CAD build for the part. Positions are in the model's coordinates, mm. A direction names the side the tool comes from. Coordinates: 2 decimals unless noted, no trailing zeros. Loops run counter-clockwise (first coordinate to the right, second up) from the corner with the lowest first, then second, coordinate; pieces in that order, holes last. Notation, with made-up numbers: (82, -19) - (116, -19) arc R25 cw to (116, 4) - close; hole circle Ø11 at (2, 49). An arc over 180 degrees is marked (long way). Put each result on its own line as item: value.
Autodesk Inventor part; units mm, degrees
ref_plane "Work Plane1" through (0, 0, -15) normal (0, 0, 1) x (1, 0, 0)
ref_plane "YZ Plane" through (0, 0, 0) normal (1, 0, 0) x (0, 1, 0)
ref_plane "XZ Plane" through (0, 0, 0) normal (0, 1, 0) x (-1, 0, 0)
sketch "Sketch1" plane through (0, 0, 0) normal (0, 0, 1) x (1, 0, 0)
  line L0 (0, 0) -> (25, 0)
  line L1 (25, 0) -> (25, 40)
  line L2 (25, 40) -> (0, 40)
  line L3 (0, 40) -> (0, 0)
  dimension "d1" = 25
  dimension "d2" = 40
  dimension "d3" = 25
extrude "Extrusion1" add sketch "Sketch1" against normal blind 30
sketch "Sketch2" plane through (25, 0, 0) normal (1, 0, 0) x (0, 0, -1)
  line L0 (0, 0) -> (30, 0)
  circle A0 centre (15, 6.56) radius 2.46
extrude "Extrusion2" cut sketch "Sketch2" against normal blind 30
sketch "Sketch3" plane through (0, 0, 0) normal (-1, 0, 0) x (0, 0, 1)
  line L0 (0, 0) -> (-30, 0)
  line L1 (-25.05, 0) -> (-4.95, 0)
  line L2 (-4.95, 0) -> (-4.95, 33.12)
  line L3 (-4.95, 33.12) -> (-25.05, 33.12)
  line L4 (-25.05, 33.12) -> (-25.05, 0)
  dimension "d11" = 20.1
extrude "Extrusion3" cut sketch "Sketch3" against normal blind 20
sketch "Sketch4" plane through (0, 0, 0) normal (0, -1, 0) x (1, 0, 0)
  line L0 (20, -4.95) -> (20, -25.05)
  line L1 (20, -15) -> (25, -15)
  line L2 (25, 0) -> (25, -30)
  line L3 (20, -8.025) -> (25, -8.025)
  line L4 (25, -8.025) -> (25, -21.975)
  line L5 (25, -21.975) -> (20, -21.975)
  line L6 (20, -21.975) -> (20, -8.025)
  line L7 (20, -8.025) -> (25, -21.975) construction
  line L8 (25, -8.025) -> (20, -21.975) construction
  line L9 (25, -12.54) -> (25, -17.46)
  point P0 (0, 0)
  point P1 (22.5, -15)
  dimension "d14" = 13.95
extrude "Extrusion4" add sketch "Sketch4" along normal blind 15
sketch "Sketch5" plane through (20, 0, 0) normal (-1, 0, 0) x (0, 0, 1)
  circle A0 centre (-15, 6.56) radius 2.46
  circle A1 centre (-15, 6.56) radius 4.7025
  circle A2 centre (-15, 6.56) radius 2.46
  circle A3 centre (-15, 6.56) radius 2.46
  point P0 (0, 0)
  dimension "d17" = 9.405
extrude "Extrusion5" cut sketch "Sketch5" against normal blind 2.1
sketch "Sketch6" plane through (25, 0, 0) normal (1, 0, 0) x (0, 0, -1)
  circle A0 centre (15, 6.56) radius 4.7025
  line L0 (15, 6.56) -> (15, 23.56)
  circle A1 centre (15, 23.56) radius 2.46
  point P0 (0, 0)
  dimension "d20" = 17
  dimension "d21" = 4.92
extrude "Extrusion6" cut sketch "Sketch6" against normal blind 10 contours A1
sketch "Sketch7" plane through (20, 0, 0) normal (-1, 0, 0) x (0, 0, 1)
  circle A0 centre (-15, 23.56) radius 2.46
  circle A1 centre (-15, 23.56) radius 4.7025
  point P0 (0, 0)
  dimension "d24" = 9.405
extrude "Extrusion7" cut sketch "Sketch7" against normal blind 2.1
sketch "Sketch9" plane through (25, 0, 0) normal (1, 0, 0) x (0, 0, -1)
  circle A0 centre (15, 6.56) radius 2.46
  circle A1 centre (15, 6.56) radius 2.46
  circle A2 centre (15, 23.56) radius 2.46
  circle A3 centre (15, 23.56) radius 2.46
  line L0 (30, 40) -> (30, 0)
  line L1 (30, 0) -> (30, 40)
  line L2 (30, 40) -> (0, 40)
  line L3 (0, 40) -> (0, 0)
  line L4 (0, 0) -> (8.025, 0)
  line L5 (21.975, 0) -> (21.975, -15)
  line L6 (21.975, -15) -> (8.025, -15)
  line L7 (8.025, -15) -> (8.025, 0)
  line L8 (0, 0) -> (8.025, 0)
  line L9 (21.975, 0) -> (30, 0)
extrude "Extrusion8" add sketch "Sketch9" along normal blind 5
sketch "Sketch10" plane through (0, 40, 0) normal (0, 1, 0) x (1, 0, 0)
  line L0 (0, 30) -> (30, 30)
  line L1 (30, 0) -> (0, 0)
  line L2 (0, 30) -> (30, 30)
  line L3 (30, 30) -> (30, 0)
  line L4 (30, 0) -> (0, 0)
  line L5 (0, 0) -> (0, 30)
extrude "Extrusion9" add sketch "Sketch10" along normal blind 30
sketch "Sketch12" plane through (30, 0, 0) normal (1, 0, 0) x (0, 0, -1)
  circle A0 centre (15, 6.56) radius 2.46
  line L0 (15, 6.56) -> (15, 15.06)
  circle A1 centre (15, 15.06) radius 2.525
  point P0 (0, 0)
  dimension "d31" = 8.5
  dimension "d33" = 5.05
extrude "Extrusion10" cut sketch "Sketch12" against normal blind 30 contours A1
sketch "Sketch14" plane through (0, 0, 0) normal (0, 0, 1) x (1, 0, 0)
  line L0 (30, 70) -> (0, 70)
  line L1 (0, 70) -> (0, 85)
  line L2 (30, 0) -> (30, 70)
  line L3 (30, 118) -> (30, 70)
  line L4 (30, 105) -> (30, 100)
  line L5 (-7, 134) -> (-12, 136)
  line L6 (-7, 102) -> (-12, 100)
  line L7 (-7, 102) -> (-2, 118)
  line L8 (-2, 118) -> (-7, 134)
  line L9 (15, 136) -> (30, 118)
  line L10 (-12, 136) -> (15, 136)
  line L11 (0, 85) -> (0, 100)
  line L12 (0, 100) -> (-12, 100)
  point P0 (0, 0)
  dimension "d82" = 12
extrude "Extrusion12" add sketch "Sketch14" against normal blind 30
sketch "Sketch15" plane through (0, 0, -25.05) normal (-1, 0, 0) x (0, 0, 1)
  line L0 (0, 33.12) -> (20.1, 33.12)
  line L1 (20.1, 33.12) -> (20.1, 0)
  line L2 (0, 33.12) -> (20.1, 33.12)
  line L3 (20.1, 33.12) -> (20.1, 31.1)
  line L4 (20.1, 31.1) -> (0, 31.1)
  line L5 (0, 31.1) -> (0, 33.12)
  point P0 (25.05, 0)
  dimension "d57" = 2.02
extrude "Extrusion13" add sketch "Sketch15" against normal blind 20
sketch "Sketch23" plane through (0, 0, 0) normal (0, 0, 1) x (1, 0, 0)
  line L0 (0, 100) -> (-12, 100)
  line L1 (0, 100) -> (-12, 100)
  line L2 (-12, 100) -> (-7, 102)
  line L3 (-12, 100) -> (-7, 102)
  line L4 (-7, 102) -> (-2, 118)
  line L5 (-7, 102) -> (-2, 118)
  line L6 (-2, 118) -> (-7, 134)
  line L7 (-2, 118) -> (-7, 134)
  line L8 (-12, 136) -> (15, 136)
  line L9 (-7, 134) -> (-12, 136)
  line L10 (-12, 136) -> (15, 136)
  line L11 (15, 136) -> (30, 118)
  line L12 (15, 136) -> (30, 118)
  line L13 (30, 118) -> (30, 88)
  line L14 (30, 0) -> (30, 118)
  line L15 (30, 88) -> (0, 88)
  line L16 (0, 88) -> (0, 100)
  point P0 (0, 0)
  dimension "d83" = 30
  dimension "d84" = 30
extrude "Extrusion14" add sketch "Sketch23" along normal blind 15
ref_plane "Work Plane1" through (0, 0, -15) normal (0, 0, 1) x (1, 0, 0)
mirror "Mirror1" about plane through (0, 0, -15) normal (0, 0, 1) of "Extrusion14"
properties part number "rec_b_32mm_x_60mm"
Q1. Wall check: L1, parallel to Z at x = 21, y = 23; L2, parallel to Z at x = 0.5, y = 8; L3, parallel to Y at x = 26.75, z = -15 (3 decimals). Give the ranges that are in metal, low to high. Write a range as from..to.
Determined:
L1: -30..-19.67, -10.33..0
L2: -30..-25.05, -4.95..0
L3: -15..4.1, 9.02..12.535, 17.585..21.1, 26.02..121.9
Q2. Slice it at A-A, the plane y = 15.06. Give the cut face in (x, z) (3 decimals).
Determined:
outline: (0, -30) - (30, -30) - (30, -17.525) - (20, -17.525) - (20, -25.05) - (0, -25.05) - close; (0, -4.95) - (20, -4.95) - (20, -12.475) - (30, -12.475) - (30, 0) - (0, 0) - close
Q3. Mould opens along Z. For faces 1 (the flat face through (14, 112, -45)), 2 (the flat face through (-4.465, 110.112, -14.58)), 3 (the flat face through (22.1, 4.5, -13)), 4 (the flat face through (13, 112, 15)) say: +Z half, -Z half, draft (parallel to the pull), parting line (faces both ways), or undercut.
Determined:
face 1: -Z half
face 2: draft
face 3: undercut
face 4: +Z half
Q4. Pin check, flat tips, straight feed: pin 1 Ø12 at (y, z) = (6.56, -15) entering from -X; pin 2 Ø5 at (x, y) = (27, -9) entering from +Z (3 decimals); pin 3 Ø5 at (x, z) = (-2, -34) entering from -Y; pin 4 Ø4.5 at (y, z) = (15.06, -15) entering from +X. Stop position of each tip, or through.
Determined:
pin 1: x = 20
pin 2: z = -8.025
pin 3: y = 88
pin 4: through
Q5. Tool access for faces 5 (the flat face through (-4.535, 126.112, -14.58)), 6 (the flat face through (10, 16, -25.05)), 7 (the flat face through (15, 88, 7)), 8 (the flat face through (25, -7, -21.975)): list every direction of +Z, -Z, +X, -X, +Y, -Y with a clear straight run to the whole face (end or side of a thin tool).
Determined:
face 5: +Z, -Z, -X
face 6: -X, -Y
face 7: +Z, +X, -X, -Y
face 8: -Z, +X, -X, -Y
Q6. Slice it at D-D, the plane z = 10. Give the cut face in (x, y).
Determined:
outline: (-12, 100) - (0, 100) - (0, 88) - (30, 88) - (30, 118) - (15, 136) - (-12, 136) - (-7, 134) - (-2, 118) - (-7, 102) - close
Q7. Slice it at B-B, the plane x = 27.5. Give the cut face in (y, z) (3 decimals).
Determined:
outline: (-15, -21.975) - (0, -21.975) - (0, -30) - (88, -30) - (88, -45) - (121, -45) - (121, 15) - (88, 15) - (88, 0) - (0, 0) - (0, -8.025) - (-15, -8.025) - close; hole circle Ø4.92 at (6.56, -15); hole circle Ø5.05 at (15.06, -15); hole circle Ø4.92 at (23.56, -15)
Q8. Slice it at C-C, the plane z = -15. State how many separate pieces and enclosed holes the cut face has, then the cut area to 3 significant figures.
Determined:
separate pieces: 4
enclosed holes: 0
area: 3,490 mm2
